Geometry check sheet. Reference: the model listing, model coordinates, mm. Face numbers are marked on the shaded views. A direction names the side the tool comes from. Give positions to 0.01 mm unless a question says otherwise; leave off trailing zeros. Write each loop counter-clockwise with the first axis right and the second up, starting at its lowest first coordinate (ties: lowest second). Pieces come first, ordered by that corner, then holes. Notation, with made-up numbers: (-24, 3) - (35, 3) arc R35 cw to (35, 36) - close; hole circle Ø7 at (-7, 51.25). An arc over 180 degrees is marked (long way). Use a Markdown table: item, result.
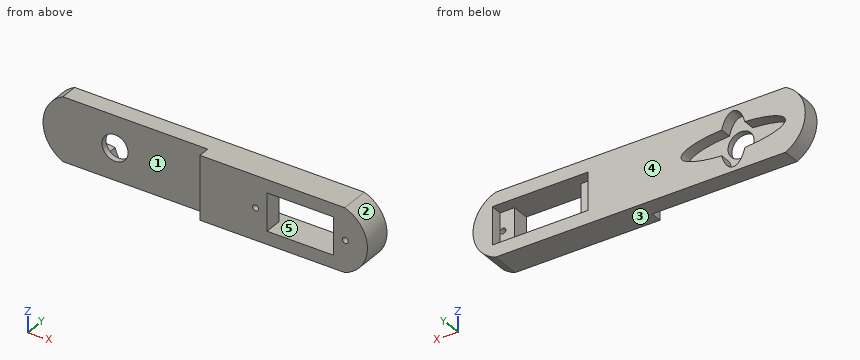
```python
from build123d import *

# Parameters (mm, degrees)
EXTRUDE_1_DEPTH     = 10
SKETCH_2_R          = 4.5
CUT_EXTRUDE_1_DEPTH = 21
CUT_EXTRUDE_2_DEPTH = 4
SKETCH_4_W          = 23
SKETCH_4_H          = 13
CUT_EXTRUDE_3_DEPTH = 21
SKETCH_5_W          = 5
SKETCH_5_H          = 13
CUT_EXTRUDE_4_DEPTH = 4
CUT_EXTRUDE_5_DEPTH = 10
SKETCH_7_R          = 1
CUT_EXTRUDE_6_DEPTH = 11
CUT_EXTRUDE_7_DEPTH = 4


with BuildPart() as part:
    # 草图1 → 凸台-拉伸1 (new body, symmetric)
    with BuildSketch(Plane(origin=(0, 0, 0), x_dir=(1, 0, 0), z_dir=(0, 1, 0))):
        with BuildLine():
            Line((-18, 11), (82, 11))
            ThreePointArc((82, 11), (89.822046697, 0), (82, -11))
            Line((82, -11), (-18, -11))
            ThreePointArc((-18, -11), (-24.855224852, 0), (-18, 11))
        make_face()
    extrude(amount=EXTRUDE_1_DEPTH, both=True)

    # 草图2 → 切除-拉伸1 (cut, through all)
    with BuildSketch(Plane(origin=(0, 10, 0), x_dir=(1, 0, 0), z_dir=(0, 1, 0))):
        Circle(SKETCH_2_R)
    extrude(amount=-CUT_EXTRUDE_1_DEPTH, mode=Mode.SUBTRACT)

    # 草图3 → 切除-拉伸2 (cut)
    with BuildSketch(Plane(origin=(0, 10, 0), x_dir=(1, 0, 0), z_dir=(0, 1, 0))):
        with BuildLine():
            add(Edge.make_bspline(
                [(-3.991210712, 4.387982431), (-18, 3.591602336), (-18, 0), (-18, -3.591602336), (-3.991210712, -4.387982431)],
                knots=[1.794388632, 1.794388632, 1.794388632, 3.141592654, 3.141592654, 4.488796676, 4.488796676, 4.488796676], degree=2, weights=[1, 0.781579788, 1, 0.781579788, 1]))
            add(Edge.make_bspline(
                [(-3.991210712, -4.387982431), (0, -20.567539049), (3.991210712, -4.387982431)],
                knots=[2.05092453, 2.05092453, 2.05092453, 4.232260777, 4.232260777, 4.232260777], degree=2, weights=[1, 0.461892887, 1]))
            add(Edge.make_bspline(
                [(3.991210712, -4.387982431), (18, -3.591602336), (18, 0), (18, 3.591602336), (3.991210712, 4.387982431)],
                knots=[4.935981285, 4.935981285, 4.935981285, 6.283185307, 6.283185307, 7.630389329, 7.630389329, 7.630389329], degree=2, weights=[1, 0.781579788, 1, 0.781579788, 1]))
            add(Edge.make_bspline(
                [(3.991210712, 4.387982431), (0, 20.567539049), (-3.991210712, 4.387982431)],
                knots=[5.192517184, 5.192517184, 5.192517184, 7.373853431, 7.373853431, 7.373853431], degree=2, weights=[1, 0.461892887, 1]))
        make_face()
    extrude(amount=-CUT_EXTRUDE_2_DEPTH, mode=Mode.SUBTRACT)

    # 草图4 → 切除-拉伸3 (cut, through all)
    with BuildSketch(Plane(origin=(0, 10, 0), x_dir=(1, 0, 0), z_dir=(0, 1, 0))):
        with Locations((66.67647479, 0)):
            Rectangle(SKETCH_4_W, SKETCH_4_H)
    extrude(amount=-CUT_EXTRUDE_3_DEPTH, mode=Mode.SUBTRACT)

    # 草图5 → 切除-拉伸4 (cut)
    with BuildSketch(Plane(origin=(0, 10, 0), x_dir=(1, 0, 0), z_dir=(0, 1, 0))):
        with Locations((52.67647479, 0)):
            Rectangle(SKETCH_5_W, SKETCH_5_H)
        with Locations((80.67647479, 0)):
            Rectangle(SKETCH_5_W, SKETCH_5_H)
    extrude(amount=-CUT_EXTRUDE_4_DEPTH, mode=Mode.SUBTRACT)

    # 草图6 → 切除-拉伸5 (cut)
    with BuildSketch(Plane(origin=(0, -10, 0), x_dir=(-1, 0, 0), z_dir=(0, -1, 0))):
        with BuildLine():
            Line((18, 11), (-82, 11))
            ThreePointArc((-82, 11), (-89.822046697, 0), (-82, -11))
            Line((-82, -11), (18, -11))
            ThreePointArc((18, -11), (24.855224852, 0), (18, 11))
        make_face()
    extrude(amount=-CUT_EXTRUDE_5_DEPTH, mode=Mode.SUBTRACT)

    # 草图7 → 切除-拉伸6 (cut, through all)
    with BuildSketch(Plane(origin=(0, 10, 0), x_dir=(1, 0, 0), z_dir=(0, 1, 0))):
        with Locations((82.17647479, 0)):
            Circle(SKETCH_7_R)
        with Locations((51.17647479, 0)):
            Circle(SKETCH_7_R)
    extrude(amount=-CUT_EXTRUDE_6_DEPTH, mode=Mode.SUBTRACT)

    # 草图8 → 切除-拉伸7 (cut)
    with BuildSketch(Plane(origin=(0, 0, 0), x_dir=(-1, 0, 0), z_dir=(0, -1, 0))):
        with BuildLine():
            Line((-32, -11), (18, -11))
            ThreePointArc((18, -11), (24.855224852, 0), (18, 11))
            Line((18, 11), (-32, 11))
            Line((-32, 11), (-32, -11))
        make_face()
    extrude(amount=-CUT_EXTRUDE_7_DEPTH, mode=Mode.SUBTRACT)


solid = part.part
```
1) Section check B-B on y = 1.75. Record the boundary of the cut face in (x, z), then the cut area to 3 significant figures.
Working result:
| item | result |
|---|---|
| outline | (32, -11) - (82, -11) arc R11.65 ccw to (82, 11) - (32, 11) - close; hole circle Ø2 at (51.18, 0); hole (55.18, -6.5) - (78.18, -6.5) - (78.18, 6.5) - (55.18, 6.5) - close; hole circle Ø2 at (82.18, 0) |
| area | 920 mm² |
2) Section check C-C on y = 9. Count the separate pieces of the cut face and the enclosed holes in it, then the cut area to 3 significant figures.
Working result:
| item | result |
|---|---|
| separate pieces | 1 |
| enclosed holes | 2 |
| area | 1,690 mm² |
3) Mould release check, pull along Z, two halves, no side actions. Record for the marked faces 3, 4 and 5: pulls with the +Z half, pulls with the -Z half, needs draft (parallel to the pull), parting line crosses it, or undercut.
Working result:
| item | result |
|---|---|
| face 3 | pulls with the -Z half |
| face 4 | needs draft |
| face 5 | undercut |
4) Depth check by flat-ended pin: P1, Ø1.2, axis at y = 8.5, z = 3, coming from the -X side; P2, Ø5, axis at x = 53, z = -1, coming from the +Y side; P3, Ø6, axis at x = 7.5, z = 5.5, coming from the -Y side. Enter the tip coordinate at first touch or a pass-through.
Working result:
| item | result |
|---|---|
| P1 | stops at x = -24.62 |
| P2 | stops at y = 6 |
| P3 | stops at y = 4 |
5) Section check A-A on x = 67. Record the boundary of the cut face in (y, z).
Working result:
| item | result |
|---|---|
| outline | (0, -11) - (10, -11) - (10, -6.5) - (0, -6.5) - close; (0, 6.5) - (10, 6.5) - (10, 11) - (0, 11) - close |
6) Set-up check for the marked faces 1 and 2: record each of +Z, -Z, +X, -X, +Y, -Y from which the full face is reachable in a straight line by a thin tool's end or side.
Working result:
| item | result |
|---|---|
| face 1 | +Z, -Z, -X, -Y |
| face 2 | +X, +Y, -Y |
7) Material ranges on L1, parallel to X at y = 4.5, z = 0; L2, parallel to X at y = 2.6, z = 0; L3, parallel to Z at x = 58.5, y = 5.75, recorded low to high. Write a range as from..to.
Working result:
| item | result |
|---|---|
| L1 | x = -24.86..-4.5, 4.5..50.18, 52.18..55.18, 78.18..81.18, 83.18..89.82 |
| L2 | x = 32..50.18, 52.18..55.18, 78.18..81.18, 83.18..89.82 |
| L3 | z = -11..-6.5, 6.5..11 |
